Answer from the drawing. Dimensions are ordinates in mm from the lowest x, y and z of the part. Give positions to 0.01 mm unless a question says otherwise; leave off trailing zeros. Order: outer loops, then holes, each group sorted by start corner. A loop starts at its lowest first (then second) coordinate and runs counter-clockwise, first axis right, second up. Notation, with made-up numbers: (81, 64.5) - (111, 64.5) arc R8 ccw to (111, 69.5) - close; hole circle Ø8 at (-6.5, -14.75). An arc over 180 degrees is marked (long way). One line per item, written item: value. Start each with the question number.
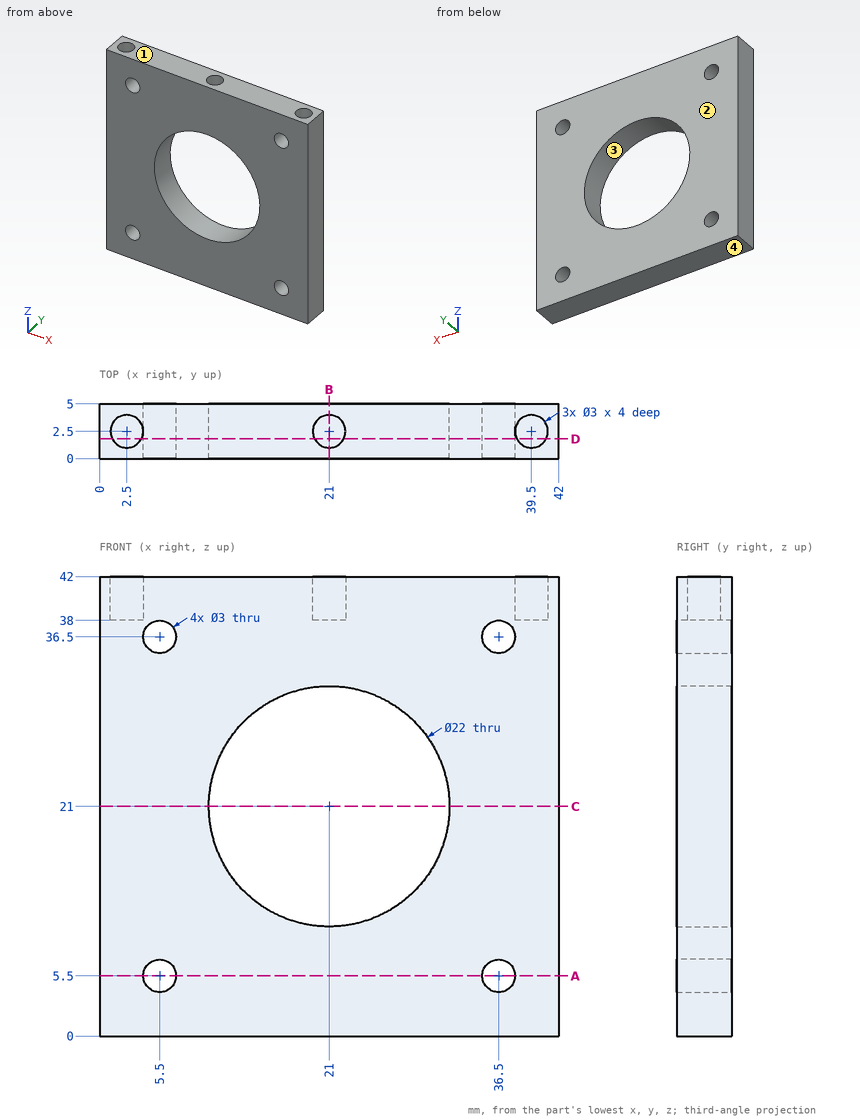
1) The mould has two halves that part along Z. Classify the marked faces 1, 2, 3 and 4: +Z half, -Z half, draft (parallel to the pull), parting line (faces both ways), or undercut.
2) Each of these flat-tipped pins is pushed along its axis until it touches: pin 1 (4 mm diameter, centred on x = 5.5, z = 36.5, fed in from -Y); pin 2 (10 mm diameter, centred on x = 17, z = 17, fed in from -Y); pin 3 (0.9 mm diameter, centred on x = 2.5, y = 2, fed in from +Z). Where does it stop, or does it pass through?
3) Section B-B on x = 21 is taken. Write down the section's boundary in (y, z).
4) Find the intervals of material crossed by probe 1 along Z at (x, y) = (36.5, 2.85); probe 2 along Y at (x, z) = (39.5, 40.9), in increasing order. Write a range as from..to.
5) Section C-C on z = 21 is taken. Write down the section's boundary in (x, y), plus the area to 3 significant figures.
6) Section D-D on y = 1.8 is taken. Write down the section's boundary in (x, z), plus the area to 3 significant figures.
7) Section A-A on z = 5.5 is taken. Write down the section's boundary in (x, y).
Solved:
1. face 1: +Z half
1. face 2: draft
1. face 3: undercut
1. face 4: -Z half
2. pin 1: stops at y = 0
2. pin 2: passes through
2. pin 3: stops at z = 38
3. outline: (0, 0) - (5, 0) - (5, 10) - (0, 10) - close; (0, 32) - (5, 32) - (5, 42) - (4, 42) - (4, 38) - (1, 38) - (1, 42) - (0, 42) - close
4. probe 1: z = 0..4, 7..35, 38..42
4. probe 2: y = 0..1, 4..5
5. outline: (0, 0) - (10, 0) - (10, 5) - (0, 5) - close; (32, 0) - (42, 0) - (42, 5) - (32, 5) - close
5. area: 100 mm2
6. outline: (0, 0) - (42, 0) - (42, 42) - (40.83, 42) - (40.83, 38) - (38.17, 38) - (38.17, 42) - (22.33, 42) - (22.33, 38) - (19.67, 38) - (19.67, 42) - (3.83, 42) - (3.83, 38) - (1.17, 38) - (1.17, 42) - (0, 42) - close; hole circle Ø3 at (5.5, 5.5); hole circle Ø3 at (5.5, 36.5); hole circle Ø22 at (21, 21); hole circle Ø3 at (36.5, 5.5); hole circle Ø3 at (36.5, 36.5)
6. area: 1,320 mm2
7. outline: (0, 0) - (4, 0) - (4, 5) - (0, 5) - close; (7, 0) - (35, 0) - (35, 5) - (7, 5) - close; (38, 0) - (42, 0) - (42, 5) - (38, 5) - close
